Model file for the job. Use its own axes, mm. Face numbers are marked on the shaded views. Give positions to 0.01 mm unless a question says otherwise; leave off trailing zeros. Order: outer loops, then holes, each group sorted by start corner. A loop starts at its lowest first (then second) coordinate and runs counter-clockwise, first axis right, second up. Notation, with made-up numbers: (67, -0.5) -> (126, -0.5) arc R19 ccw to (126, 5.5) -> close; hole circle Ø5 at (75.5, 9). An arc over 180 degrees is marked (long way). Use CSV: the item, a comma, the result in double quotes. Start each with the question number.
1. Cut at C-C on y = 0.1. List the corners of the cut face in (x, z), then the cut area to 3 significant figures.
2. Cut at A-A on x = 0. List the corners of the cut face in (y, z), then the cut area to 3 significant figures.
3. Drop flat-ended pins along their axis: pin 1 (1.5 mm diameter, centred on y = -1, z = -3.5, fed in from +X); pin 2 (1 mm diameter, centred on x = 10.5, y = 0.5, fed in from -Z); pin 3 (1.5 mm diameter, centred on x = 3.5, y = 1, fed in from +Z). Give the stop position or say it passes through.
4. Pull direction Z, two halves, no side cores. Call the marked faces 1, 2 and 3: released by +Z, released by -Z, zero draft, split by the parting line, or undercut.
5. Cut at B-B on z = 0. List the corners of the cut face in (x, y), then the cut area to 3 significant figures.
6. Wall check: line 1 (Z direction, x = 0, y = 0.9); line 2 (X direction, y = 0.8, z = -9.5); line 3 (X direction, y = -0.7, z = -11). Give the ranges that are in metal, low to high. Write a range as from..to.
7. Cut at D-D on z = -9.5. List the corners of the cut face in (x, y), then the cut area to 3 significant figures.
Solid Edge part; units mm, degrees
sketch "Sketch1" plane through (0, 0, 0) normal (0, -1, 0) x (1, 0, 0)
  circle A0 centre (0, 0) radius 17.5
extrude "Protrusion1" add sketch "Sketch1" along normal mid plane 3
sketch "Sketch2" plane through (0, -1.5, 0) normal (0, -1, 0) x (1, 0, 0)
  line L0 (-1.4832, 0.6) -> (1.4832, 0.6)
  arc A0 (1.4832, 0.6) -> (-1.4832, 0.6) centre (0, 0) cw
extrude "Cutout1" cut sketch "Sketch2" against normal up to vertex (3 mm away)
hole "Agujero_1" at (0, -1.5, 9.98) direction (0, 1, 0) diameter 3.2 end up to next
pattern_circular "Pattern1" count 4 over 360 about axis through (0, -1.5, 0) along (0, 1, 0) of "Agujero_1"
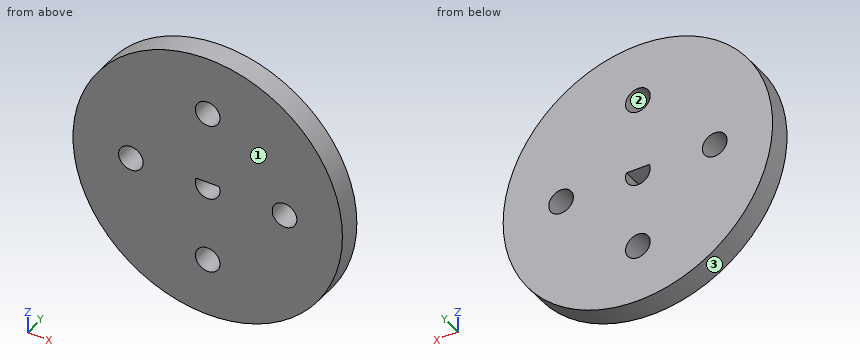
Verdict:
1,outline,"circle Ø35 at (0, 0); hole circle Ø3.2 at (-9.98, 0); hole circle Ø3.2 at (0, -9.98); hole circle Ø3.2 at (0, 9.98); hole (-1.48, 0.6) arc R1.6 ccw (long way) to (1.48, 0.6) -> close; hole circle Ø3.2 at (9.98, 0)"
1,area,"924 mm^2"
2,outline,"(-1.5, -17.5) -> (1.5, -17.5) -> (1.5, -11.58) -> (-1.5, -11.58) -> close; (-1.5, -8.38) -> (1.5, -8.38) -> (1.5, -1.6) -> (-1.5, -1.6) -> close; (-1.5, 0.6) -> (1.5, 0.6) -> (1.5, 8.38) -> (-1.5, 8.38) -> close; (-1.5, 11.58) -> (1.5, 11.58) -> (1.5, 17.5) -> (-1.5, 17.5) -> close"
2,area,"79.2 mm^2"
3,pin 1,"x = 17.28"
3,pin 2,"z = -14.36"
3,pin 3,"z = 17.28"
4,face 1,"zero draft"
4,face 2,"undercut"
4,face 3,"split by the parting line"
5,outline,"(-17.5, -1.5) -> (-11.58, -1.5) -> (-11.58, 1.5) -> (-17.5, 1.5) -> close; (-8.38, -1.5) -> (-1.6, -1.5) -> (-1.6, 1.5) -> (-8.38, 1.5) -> close; (1.6, -1.5) -> (8.38, -1.5) -> (8.38, 1.5) -> (1.6, 1.5) -> close; (11.58, -1.5) -> (17.5, -1.5) -> (17.5, 1.5) -> (11.58, 1.5) -> close"
5,area,"76.2 mm^2"
6,line 1,"-17.5..-11.58, -8.38..-1.6, 0.6..8.38, 11.58..17.5"
6,line 2,"-14.7..-1.53, 1.53..14.7"
6,line 3,"-13.61..-1.23, 1.23..13.61"
7,outline,"(-14.7, -1.5) -> (-1.53, -1.5) -> (-1.53, 1.5) -> (-14.7, 1.5) -> close; (1.53, -1.5) -> (14.7, -1.5) -> (14.7, 1.5) -> (1.53, 1.5) -> close"
7,area,"79.0 mm^2"
